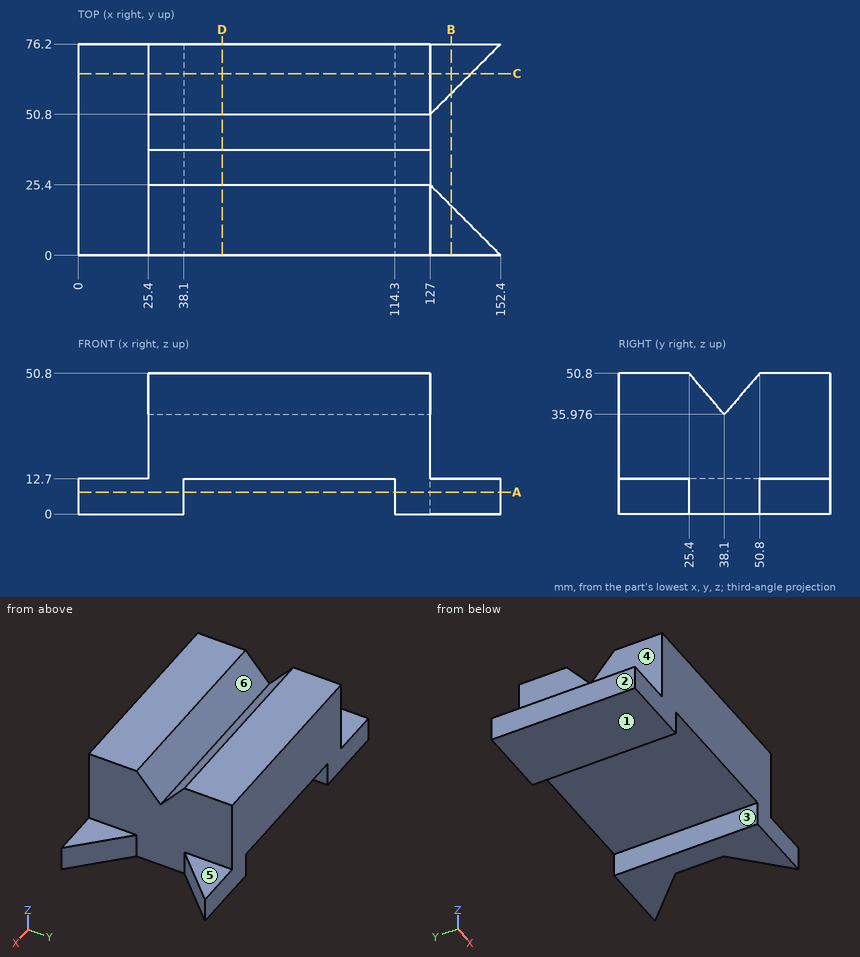
Could you check a few things on this drawing? It's one solid part, dimensions in mm from its lowest x, y, z. A direction names the side the tool comes from. Coordinates: 2 decimals unless noted, no trailing zeros. Write each loop counter-clockwise with the first axis right and the second up, starting at its lowest first coordinate (ties: lowest second). Pieces come first, ordered by that corner, then holes. Notation, with made-up numbers: (-35, 52.25) - (-30, 52.25) arc R14 ccw to (-30, 57.25) - close; hole circle Ø10 at (-27.5, 17.25). An arc over 180 degrees is marked (long way). Use one line per item in the form item = value.
1) Thinking about a two-plate mould opening in X: for the marked faces 1, 2 and 3, which applies, released by +X, released by -X, zero draft, split by the parting line, or undercut?
Solved:
face_1 = zero draft
face_2 = released by -X
face_3 = undercut
2) Suppose I cut it at B-B, the plane x = 134.5. Write out the boundary of the cut face in (y, z), plus the area to 3 significant figures.
Solved:
outline = (0, 0) - (17.9, 0) - (17.9, 12.7) - (0, 12.7) - close; (58.3, 0) - (76.2, 0) - (76.2, 12.7) - (58.3, 12.7) - close
area = 455 mm2
3) On a 3-axis mill with a long thin cutter (end or side, diameter ignored), from which of +Z, -Z, +X, -X, +Y, -Y can I reach the whole of each face in a straight line? I mean the marked faces 4, 5 and 6. Say none if no direction works.
Solved:
face_4 = +Z, -X, +Y, -Y
face_5 = +Z, +X, +Y, -Y
face_6 = +Z, +X, -X
4) Suppose I cut it at A-A, the plane z = 8. Write out the boundary of the cut face in (x, y), plus the area to 3 significant figures.
Solved:
outline = (0, 0) - (38.1, 0) - (38.1, 76.2) - (0, 76.2) - close; (114.3, 0) - (152.4, 0) - (127, 25.4) - (127, 50.8) - (152.4, 76.2) - (114.3, 76.2) - close
area = 4,520 mm2
5) I'm going to push flat-ended pins straight in: P1, Ø11.5, axis at y = 52.5, z = 35.5, coming from the -X side; P2, Ø6.5, axis at y = 36.5, z = 4.5, coming from the +X side; P3, Ø20.5, axis at x = 18, y = 31, coming from the +Z side; P4, Ø7.5, axis at x = 137, y = 13.5, coming from the +Z side. Where does each tip first touch, or does it pass through?
Solved:
P1 = 25.4
P2 = 127
P3 = 50.8
P4 = 12.7
6) Suppose I cut it at C-C, the plane y = 65.5. Write out the boundary of the cut face in (x, z).
Solved:
outline = (0, 0) - (38.1, 0) - (38.1, 12.7) - (114.3, 12.7) - (114.3, 0) - (141.7, 0) - (141.7, 12.7) - (127, 12.7) - (127, 50.8) - (25.4, 50.8) - (25.4, 12.7) - (0, 12.7) - close
7) Suppose I cut it at D-D, the plane x = 52. Write out the boundary of the cut face in (y, z), plus the area to 4 significant figures.
Solved:
outline = (0, 12.7) - (76.2, 12.7) - (76.2, 50.8) - (50.8, 50.8) - (38.1, 35.98) - (25.4, 50.8) - (0, 50.8) - close
area = 2,715 mm2
8) I need wall thicknesses on line 1 (X direction, y = 30, z = 38.5); line 2 (Y direction, x = 103.5, z = 49.5) (1 decimal); line 3 (X direction, y = 57.5, z = 7.5). Which ranges of each line are inside material? Lowest first, please.
Solved:
line_1 = 25.4 to 127
line_2 = 0 to 26.5, 49.7 to 76.2
line_3 = 0 to 38.1, 114.3 to 133.7
